from build123d import *

# Parameters (mm, degrees)
EXTRUDE1_DEPTH = 374
EXTRUDE2_DEPTH = 17
SKETCH4_R      = 2.5
EXTRUDE3_DEPTH = 91


with BuildPart() as part:
    # Sketch1 → Extrude1 (new body)
    with BuildSketch(Plane.XY):
        with BuildLine():
            Line((-38.142101627, 26.909417684), (-25.142101627, 26.909417684))
            ThreePointArc((-25.142101627, 26.909417684), (-23.727888065, 26.323631246), (-23.142101627, 24.909417684))
            Line((-23.142101627, 24.909417684), (-23.142101627, 11.909417684))
            ThreePointArc((-23.142101627, 11.909417684), (-23.727888065, 10.495204122), (-25.142101627, 9.909417684))
            Line((-25.142101627, 9.909417684), (-38.142101627, 9.909417684))
            ThreePointArc((-38.142101627, 9.909417684), (-39.55631519, 10.495204122), (-40.142101627, 11.909417684))
            Line((-40.142101627, 11.909417684), (-40.142101627, 24.909417684))
            ThreePointArc((-40.142101627, 24.909417684), (-39.55631519, 26.323631246), (-38.142101627, 26.909417684))
        make_face()
    extrude(amount=EXTRUDE1_DEPTH)

    # Sketch2 → Extrude2 (add)
    with BuildSketch(Plane(origin=(0, 26.909417684, 0), x_dir=(1, 0, 0), z_dir=(0, 1, 0))):
        Polygon((-23.142101627, -374), (-23.142101627, -344), (-16.142101627, -344), (-16.142101627, -374), (13.357898373, -413), (13.357898373, -534), (6.357898373, -534), (6.357898373, -414), align=None)
        Polygon((-40.142101627, -374), (-40.142101627, -344), (-47.142101627, -344), (-47.142101627, -374), (-76.642101627, -413), (-76.642101627, -534), (-69.642101627, -534), (-69.642101627, -414), align=None)
    extrude(amount=-EXTRUDE2_DEPTH)

    # Sketch4 → Extrude3 (cut, through all)
    with BuildSketch(Plane(origin=(13.357898373, 0, 0), x_dir=(0, 0, -1), z_dir=(1, 0, 0))):
        with Locations((-529, 18.409417684)):
            Circle(SKETCH4_R)
        with Locations((-9, 18.409417684)):
            Circle(SKETCH4_R)
        Polygon((-529, 26.909417684), (-534, 21.909417684), (-534, 14.909417684), (-529, 9.909417684), (-529, 0), (-556.33894416, 6.720406123), (-552.141138814, 40.050556498), (-531.5, 37.450883772), align=None)
    extrude(amount=-EXTRUDE3_DEPTH, mode=Mode.SUBTRACT)


solid = part.part
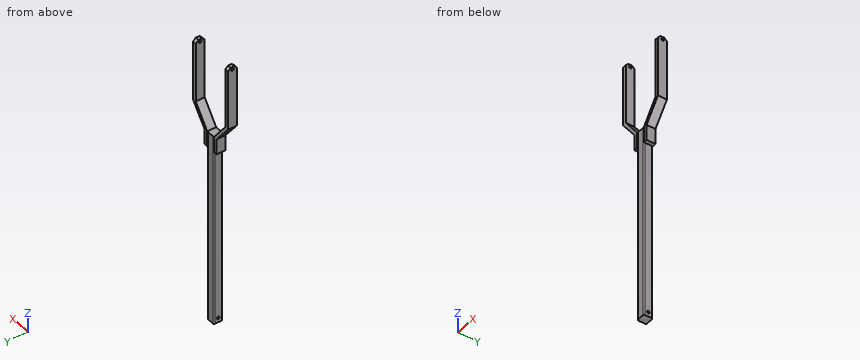
Geometry: final body of the model. Coordinates: model frame, mm. Coordinates: 2 decimals unless noted, no trailing zeros. Order: outer loops, then holes, each group sorted by start corner. A loop starts at its lowest first (then second) coordinate and runs counter-clockwise, first axis right, second up.
(1) First-contact query: pin 1 (0.6 mm diameter, centred on y = 11.5, z = 353, fed in from +X); pin 2 (5 mm diameter, centred on x = -58, y = 14.5, fed in from +Z); pin 3 (5 mm diameter, centred on x = -27, y = 15, fed in from -Z); pin 4 (1.5 mm diameter, centred on x = -63.5, y = 15.5, fed in from +Z). Flat tips, straight axial feed; report the tip coordinate or a pass-through.
(2) Material intervals for probe 1 along Y at (x, z) = (10, 529); probe 2 along X at (y, z) = (15, 466); probe 3 along X at (y, z) = (22.25, 339.5), sorted ascending.
(3) Section query A-A (z = 271). Return the cut outline in (x, y).
(4) Section query B-B (x = -57). Return the cut outline in (y, z).
Solution:
1. pin 1: stops at x = -16.14
1. pin 2: stops at z = 401.6
1. pin 3: stops at z = 0
1. pin 4: stops at z = 406.69
2. probe 1: y = 9.91 to 15.91, 20.91 to 26.91
2. probe 2: x = -76.64 to -69.64, 6.36 to 13.36
2. probe 3: x = -40.14 to -23.14
3. outline: (-40.14, 11.91) arc R2 ccw to (-38.14, 9.91) - (-25.14, 9.91) arc R2 ccw to (-23.14, 11.91) - (-23.14, 24.91) arc R2 ccw to (-25.14, 26.91) - (-38.14, 26.91) arc R2 ccw to (-40.14, 24.91) - close
4. outline: (9.91, 387.03) - (26.91, 387.03) - (26.91, 396.86) - (9.91, 396.86) - close
